Part model, mm, in its own coordinate system. A direction names the side the tool comes from. Round coordinates to 2 decimals unless told otherwise and drop trailing zeros.
1) Mould opens along Z. For faces 3 (the flat face through (173, 9, 0)), 4 (the flat face through (137, 12, -30)), 5 (the flat face through (350, 9, -130)) say: +Z half, -Z half, draft (parallel to the pull), parting line (faces both ways), or undercut.
2) Probe line 1 (X direction, y = 13.4, z = -232); line 2 (X direction, y = 6.75, z = -132); line 3 (Z direction, x = 230, y = 7). List the from-to ranges inside material, lowest first.
3) Drop flat-ended pins along their axis: P1, Ø5, axis at x = 234, z = -231, coming from the +Y side; P2, Ø4, axis at x = 230, z = -232, coming from the -Y side. Give the stop position or say it passes through.
4) 3-axis set-ups, long thin cutter, end or side, ignore diameter. For faces 1 (the flat face through (173, 18, -134)), 2 (the flat face through (133, 12, -134)): which of +Z, -Z, +X, -X, +Y, -Y reach the whole face in a straight line?
from build123d import *

# Parameters (mm, degrees)
SKETCH2_W           = 920
SKETCH2_H           = 264
BOSS_EXTRUDE1_DEPTH = 18
SKETCH1_R           = 2.5
CUT_EXTRUDE2_DEPTH  = 18
SKETCH3_R           = 8
CUT_EXTRUDE3_DEPTH  = 6
SKETCH4_W           = 570
SKETCH4_H           = 264
CUT_EXTRUDE4_DEPTH  = 20


with BuildPart() as part:
    # Sketch2 → Boss-Extrude1 (new body)
    with BuildSketch(Plane(origin=(0, 0, 0), x_dir=(1, 0, 0), z_dir=(0, 1, 0))):
        with Locations((460, 132)):
            Rectangle(SKETCH2_W, SKETCH2_H)
    extrude(amount=BOSS_EXTRUDE1_DEPTH)

    # Sketch1 → Cut-Extrude2 (cut)
    with BuildSketch(Plane(origin=(0, 18, 0), x_dir=(1, 0, 0), z_dir=(0, 1, 0))):
        with Locations(Location((40, 32, 0), (0, 0, 270))):
            Circle(SKETCH1_R)
        with Locations(Location((135, 32, 0), (0, 0, 270))):
            Circle(SKETCH1_R)
        with Locations(Location((230, 32, 0), (0, 0, 270))):
            Circle(SKETCH1_R)
        with Locations(Location((325, 32, 0), (0, 0, 270))):
            Circle(SKETCH1_R)
        with Locations(Location((420, 32, 0), (0, 0, 270))):
            Circle(SKETCH1_R)
        with Locations(Location((515, 32, 0), (0, 0, 270))):
            Circle(SKETCH1_R)
        with Locations(Location((610, 32, 0), (0, 0, 270))):
            Circle(SKETCH1_R)
        with Locations(Location((705, 32, 0), (0, 0, 270))):
            Circle(SKETCH1_R)
        with Locations(Location((800, 32, 0), (0, 0, 270))):
            Circle(SKETCH1_R)
        with Locations(Location((895, 32, 0), (0, 0, 270))):
            Circle(SKETCH1_R)
        with Locations(Location((135, 132, 0), (0, 0, 270))):
            Circle(SKETCH1_R)
        with Locations(Location((230, 132, 0), (0, 0, 270))):
            Circle(SKETCH1_R)
        with Locations(Location((325, 132, 0), (0, 0, 270))):
            Circle(SKETCH1_R)
        with Locations(Location((420, 132, 0), (0, 0, 270))):
            Circle(SKETCH1_R)
        with Locations(Location((515, 132, 0), (0, 0, 270))):
            Circle(SKETCH1_R)
        with Locations(Location((610, 132, 0), (0, 0, 270))):
            Circle(SKETCH1_R)
        with Locations(Location((705, 132, 0), (0, 0, 270))):
            Circle(SKETCH1_R)
        with Locations(Location((800, 132, 0), (0, 0, 270))):
            Circle(SKETCH1_R)
        with Locations(Location((895, 132, 0), (0, 0, 270))):
            Circle(SKETCH1_R)
        with Locations(Location((135, 232, 0), (0, 0, 270))):
            Circle(SKETCH1_R)
        with Locations(Location((230, 232, 0), (0, 0, 270))):
            Circle(SKETCH1_R)
        with Locations(Location((325, 232, 0), (0, 0, 270))):
            Circle(SKETCH1_R)
        with Locations(Location((420, 232, 0), (0, 0, 270))):
            Circle(SKETCH1_R)
        with Locations(Location((515, 232, 0), (0, 0, 270))):
            Circle(SKETCH1_R)
        with Locations(Location((610, 232, 0), (0, 0, 270))):
            Circle(SKETCH1_R)
        with Locations(Location((705, 232, 0), (0, 0, 270))):
            Circle(SKETCH1_R)
        with Locations(Location((800, 232, 0), (0, 0, 270))):
            Circle(SKETCH1_R)
        with Locations(Location((895, 232, 0), (0, 0, 270))):
            Circle(SKETCH1_R)
        with Locations(Location((40, 132, 0), (0, 0, 270))):
            Circle(SKETCH1_R)
        with Locations(Location((40, 232, 0), (0, 0, 270))):
            Circle(SKETCH1_R)
    extrude(amount=-CUT_EXTRUDE2_DEPTH, mode=Mode.SUBTRACT)

    # Sketch3 → Cut-Extrude3 (cut)
    with BuildSketch(Plane(origin=(0, 18, 0), x_dir=(1, 0, 0), z_dir=(0, 1, 0))):
        with Locations(Location((40, 32, 0), (0, 0, 270))):
            Circle(SKETCH3_R)
        with Locations(Location((135, 32, 0), (0, 0, 270))):
            Circle(SKETCH3_R)
        with Locations(Location((230, 32, 0), (0, 0, 270))):
            Circle(SKETCH3_R)
        with Locations(Location((325, 32, 0), (0, 0, 270))):
            Circle(SKETCH3_R)
        with Locations(Location((420, 32, 0), (0, 0, 270))):
            Circle(SKETCH3_R)
        with Locations(Location((515, 32, 0), (0, 0, 270))):
            Circle(SKETCH3_R)
        with Locations(Location((610, 32, 0), (0, 0, 270))):
            Circle(SKETCH3_R)
        with Locations(Location((705, 32, 0), (0, 0, 270))):
            Circle(SKETCH3_R)
        with Locations(Location((800, 32, 0), (0, 0, 270))):
            Circle(SKETCH3_R)
        with Locations(Location((895, 32, 0), (0, 0, 270))):
            Circle(SKETCH3_R)
        with Locations(Location((135, 132, 0), (0, 0, 270))):
            Circle(SKETCH3_R)
        with Locations(Location((230, 132, 0), (0, 0, 270))):
            Circle(SKETCH3_R)
        with Locations(Location((325, 132, 0), (0, 0, 270))):
            Circle(SKETCH3_R)
        with Locations(Location((420, 132, 0), (0, 0, 270))):
            Circle(SKETCH3_R)
        with Locations(Location((515, 132, 0), (0, 0, 270))):
            Circle(SKETCH3_R)
        with Locations(Location((610, 132, 0), (0, 0, 270))):
            Circle(SKETCH3_R)
        with Locations(Location((705, 132, 0), (0, 0, 270))):
            Circle(SKETCH3_R)
        with Locations(Location((800, 132, 0), (0, 0, 270))):
            Circle(SKETCH3_R)
        with Locations(Location((895, 132, 0), (0, 0, 270))):
            Circle(SKETCH3_R)
        with Locations(Location((135, 232, 0), (0, 0, 270))):
            Circle(SKETCH3_R)
        with Locations(Location((230, 232, 0), (0, 0, 270))):
            Circle(SKETCH3_R)
        with Locations(Location((325, 232, 0), (0, 0, 270))):
            Circle(SKETCH3_R)
        with Locations(Location((420, 232, 0), (0, 0, 270))):
            Circle(SKETCH3_R)
        with Locations(Location((515, 232, 0), (0, 0, 270))):
            Circle(SKETCH3_R)
        with Locations(Location((610, 232, 0), (0, 0, 270))):
            Circle(SKETCH3_R)
        with Locations(Location((705, 232, 0), (0, 0, 270))):
            Circle(SKETCH3_R)
        with Locations(Location((800, 232, 0), (0, 0, 270))):
            Circle(SKETCH3_R)
        with Locations(Location((895, 232, 0), (0, 0, 270))):
            Circle(SKETCH3_R)
        with Locations(Location((40, 132, 0), (0, 0, 270))):
            Circle(SKETCH3_R)
        with Locations(Location((40, 232, 0), (0, 0, 270))):
            Circle(SKETCH3_R)
    extrude(amount=-CUT_EXTRUDE3_DEPTH, mode=Mode.SUBTRACT)

    # Sketch4 → Cut-Extrude4 (cut)
    with BuildSketch(Plane(origin=(0, 18, 0), x_dir=(1, 0, 0), z_dir=(0, 1, 0))):
        with Locations((635, 132)):
            Rectangle(SKETCH4_W, SKETCH4_H)
    extrude(amount=-CUT_EXTRUDE4_DEPTH, mode=Mode.SUBTRACT)


solid = part.part
Reported:
1. face 3: +Z half
1. face 4: undercut
1. face 5: draft
2. line 1: x = 0 to 32, 48 to 127, 143 to 222, 238 to 317, 333 to 350
2. line 2: x = 0 to 37.5, 42.5 to 132.5, 137.5 to 227.5, 232.5 to 322.5, 327.5 to 350
2. line 3: z = -264 to -234.5, -229.5 to -134.5, -129.5 to -34.5, -29.5 to 0
3. P1: stops at y = 12
3. P2: passes through
4. face 1: +Z, -Z, +X, -X, +Y
4. face 2: +Y
